Source: CAD feature listing. Evaluate the final solid. Frame: model axes, mm. A direction names the side the tool comes from. Give positions to 0.01 mm unless a question says otherwise; leave off trailing zeros. Order: outer loops, then holes, each group sorted by start corner. A loop starts at its lowest first (then second) coordinate and runs counter-clockwise, first axis right, second up. Notation, with made-up numbers: M 35,-36.5 L 58,-36.5 A31 ccw 58,0.5 Z; hole C 24,-21 d1. An arc over 180 degrees is marked long. Use CSV: the item, a comma, the result in double quotes. Start each with the question number.
Item 1: Section query C-C on z = 10. Return loops of the section in (x, y), and give its area (3 significant figures).
Item 2: Access query for faces 4 (the face through (51, -17, 0)), 5 (the face through (63.57, -18.01, 11)), 6 (the face through (28, -10, 0)). Directions: +Z, -Z, +X, -X, +Y, -Y. A direction counts if a zero-diameter tool reaches every point of the face in a straight line with its end or side. Return the directions, or none.
Item 3: Pull-direction query (X, two-part tool) for faces 1 (the face through (29, -10, 12.5)), 2 (the face through (49.957, -17.986, -0.651)), 3 (the face through (30, -9, 0)); classes: +X half, -X half, draft (parallel to the pull), parting line (faces both ways), or undercut.
Item 4: Section query B-B on x = 45. Return loops of the section in (y, z), and give its area (3 significant figures).
Item 5: Section query D-D on x = 19. Return loops of the section in (y, z).
Item 6: First-contact query: pin 1 (4 mm diameter, centred on y = -9.5, z = -6, fed in from -X); pin 2 (1 mm diameter, centred on y = -3.5, z = 5.5, fed in from +X); pin 3 (1.5 mm diameter, centred on x = 27, z = 0.5, fed in from -Y). Flat tips, straight axial feed; report the tip coordinate or a pass-through.
Item 7: Ray query, probe 1 along X at (y, z) = (-15.75, 1); probe 2 along Y at (x, z) = (26, 11); probe 3 along X at (y, z) = (-17.6, 0). Return the intervals inside material, ascending. Write a range as from..to.
Item 8: Section query A-A on z = 0. Return loops of the section in (x, y).
from build123d import *

# Parameters (mm, degrees)
TABAN_FLAN_1_DEPTH    = 12.5
K_ELERI_START         = -19
K_ELERI_K_R1_DEPTH    = 19
IZIM2_R               = 5
KES_EKSTR_ZYON1_DEPTH = 10


# Read off the part's stored shape, not the designer's step: Köşeleri kır1
# Sheet-metal steps are written as plain solids
with BuildPart() as part:
    # Çizim1 → Taban-Flanş1 (new, symmetric)
    with BuildSketch(Plane.XY):
        with BuildLine():
            Line((0, 0), (27.2634, 0))
            ThreePointArc((27.2634, 0), (29.198468417, -0.801531583), (30, -2.7366))
            Line((30, -2.7366), (30, -16.2634))
            ThreePointArc((30, -16.2634), (30.215745145, -16.784254855), (30.7366, -17))
            Line((30.7366, -17), (65, -17))
            Line((65, -17), (65, -19))
            Line((65, -19), (30.7366, -19))
            ThreePointArc((30.7366, -19), (28.801531583, -18.198468417), (28, -16.2634))
            Line((28, -16.2634), (28, -2.7366))
            ThreePointArc((28, -2.7366), (27.784254855, -2.215745145), (27.2634, -2))
            Line((27.2634, -2), (0, -2))
            Line((0, -2), (0, 0))
        make_face()
    extrude(amount=TABAN_FLAN_1_DEPTH, both=True)

    # Köşeleri kır1 outline → Köşeleri kır1 (cut)
    with BuildSketch(Plane(origin=(0, 0, 0), x_dir=(1, 0, 0), z_dir=(0, 1, 0)).offset(K_ELERI_START)):
        with BuildLine():
            Line((0, -12.5), (5, -12.5))
            ThreePointArc((5, -12.5), (1.464466094, -11.035533906), (0, -7.5))
            Line((0, -7.5), (0, -12.5))
        make_face()
        with BuildLine():
            Line((0, 12.5), (0, 7.5))
            ThreePointArc((0, 7.5), (1.464466094, 11.035533906), (5, 12.5))
            Line((5, 12.5), (0, 12.5))
        make_face()
        with BuildLine():
            Line((65, -12.5), (65, -7.5))
            ThreePointArc((65, -7.5), (63.535533906, -11.035533906), (60, -12.5))
            Line((60, -12.5), (65, -12.5))
        make_face()
        with BuildLine():
            ThreePointArc((60, 12.5), (63.535533906, 11.035533906), (65, 7.5))
            Line((65, 7.5), (65, 12.5))
            Line((65, 12.5), (60, 12.5))
        make_face()
    extrude(amount=K_ELERI_K_R1_DEPTH, mode=Mode.SUBTRACT)

    # Çizim2 → Kes-Ekstrüzyon1 (cut)
    with BuildSketch(Plane(origin=(0, -17, 0), x_dir=(1, 0, 0), z_dir=(0, 1, 0))):
        with Locations(Location((45, 0, 0), (0, 0, 270))):
            Circle(IZIM2_R)
    extrude(amount=-KES_EKSTR_ZYON1_DEPTH, mode=Mode.SUBTRACT)


solid = part.part
Verdict:
1,outline,"M 0.67,-2 L 27.26,-2 A0.74 cw 28,-2.74 L 28,-16.26 A2.74 ccw 30.74,-19 L 64.33,-19 L 64.33,-17 L 30.74,-17 A0.74 cw 30,-16.26 L 30,-2.74 A2.74 ccw 27.26,0 L 0.67,0 Z"
1,area,"158 mm2"
2,face 4,"+Z, -Z, +X, +Y"
2,face 5,"+Z, +X, +Y, -Y"
2,face 6,"+Z, -Z, -X, -Y"
3,face 1,"draft"
3,face 2,"undercut"
3,face 3,"+X half"
4,outline,"M -19,-12.5 L -17,-12.5 L -17,-5 L -19,-5 Z; M -19,5 L -17,5 L -17,12.5 L -19,12.5 Z"
4,area,"30.0 mm2"
5,outline,"M -2,-12.5 L 0,-12.5 L 0,12.5 L -2,12.5 Z"
6,pin 1,"x = 28"
6,pin 2,"x = 30"
6,pin 3,"y = -2.18"
7,probe 1,"28..30"
7,probe 2,"-2..0"
7,probe 3,"28.35..40, 50..65"
8,outline,"M 0,-2 L 27.26,-2 A0.74 cw 28,-2.74 L 28,-16.26 A2.74 ccw 30.74,-19 L 40,-19 L 40,-17 L 30.74,-17 A0.74 cw 30,-16.26 L 30,-2.74 A2.74 ccw 27.26,0 L 0,0 Z; M 50,-19 L 65,-19 L 65,-17 L 50,-17 Z"
